For this review, use the dimensioned drawing (mm, ordinates from the lowest corner) and the shaded views. Coordinates: 2 decimals unless noted, no trailing zeros. Loops run counter-clockwise (first coordinate to the right, second up) from the corner with the lowest first, then second, coordinate; pieces in that order, holes last.
1. Take a section at A-A, the plane y = 53. State the section outline as (x, z) points.
2. Take a section at D-D, the plane x = 21. State the section outline as (y, z) points, then the cut area to 3 significant figures.
3. Take a section at B-B, the plane x = 7.5. State the section outline as (y, z) points.
4. To check wall thickness, follow probe 1 along X at (y, z) = (160, 2.1); probe 2 along Y at (x, z) = (7.5, 0.8); probe 3 along Y at (x, z) = (22, 1.8). State the ranges of each line that lie inside material, in increasing order.
5. Take a section at C-C, the plane z = 0.6. State the section outline as (x, y) points, then the cut area to 3 significant figures.
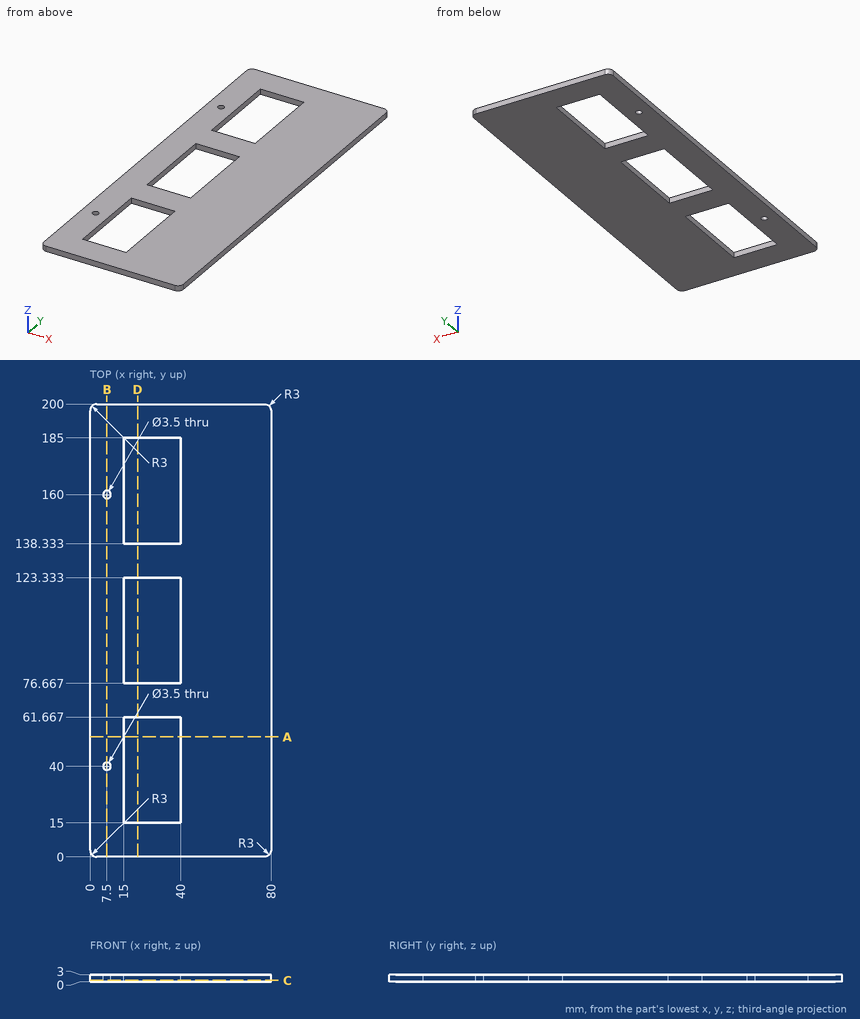
Results list:
1. outline: (0, 0) - (15, 0) - (15, 3) - (0, 3) - close; (40, 0) - (80, 0) - (80, 3) - (40, 3) - close
2. outline: (0, 0) - (15, 0) - (15, 3) - (0, 3) - close; (61.67, 0) - (76.67, 0) - (76.67, 3) - (61.67, 3) - close; (123.33, 0) - (138.33, 0) - (138.33, 3) - (123.33, 3) - close; (185, 0) - (200, 0) - (200, 3) - (185, 3) - close
2. area: 180 mm2
3. outline: (0, 0) - (38.25, 0) - (38.25, 3) - (0, 3) - close; (41.75, 0) - (158.25, 0) - (158.25, 3) - (41.75, 3) - close; (161.75, 0) - (200, 0) - (200, 3) - (161.75, 3) - close
4. probe 1: x = 0 to 5.75, 9.25 to 15, 40 to 80
4. probe 2: y = 0 to 38.25, 41.75 to 158.25, 161.75 to 200
4. probe 3: y = 0 to 15, 61.67 to 76.67, 123.33 to 138.33, 185 to 200
5. outline: (0, 3) arc R3 ccw to (3, 0) - (77, 0) arc R3 ccw to (80, 3) - (80, 197) arc R3 ccw to (77, 200) - (3, 200) arc R3 ccw to (0, 197) - close; hole circle Ø3.5 at (7.5, 40); hole circle Ø3.5 at (7.5, 160); hole (15, 15) - (40, 15) - (40, 61.67) - (15, 61.67) - close; hole (15, 76.67) - (40, 76.67) - (40, 123.33) - (15, 123.33) - close; hole (15, 138.33) - (40, 138.33) - (40, 185) - (15, 185) - close
5. area: 12,500 mm2
